Input: dimensioned drawing with shaded views. Units: mm. Origin: part minimum x, y, z. A direction names the side the tool comes from. Give positions to 0.01 mm unless a question says otherwise; leave off trailing zeros. Order: outer loops, then holes, each group sorted by start corner. A loop starts at its lowest first (then second) coordinate and runs counter-clockwise, first axis right, second up. Notation, with made-up numbers: (6, 11.5) - (16, 11.5) arc R29 cw to (16, 34.5) - close; hole circle Ø7 at (7.5, 47.25). An arc over 180 degrees is marked (long way). Answer as CSV lines item,"result".
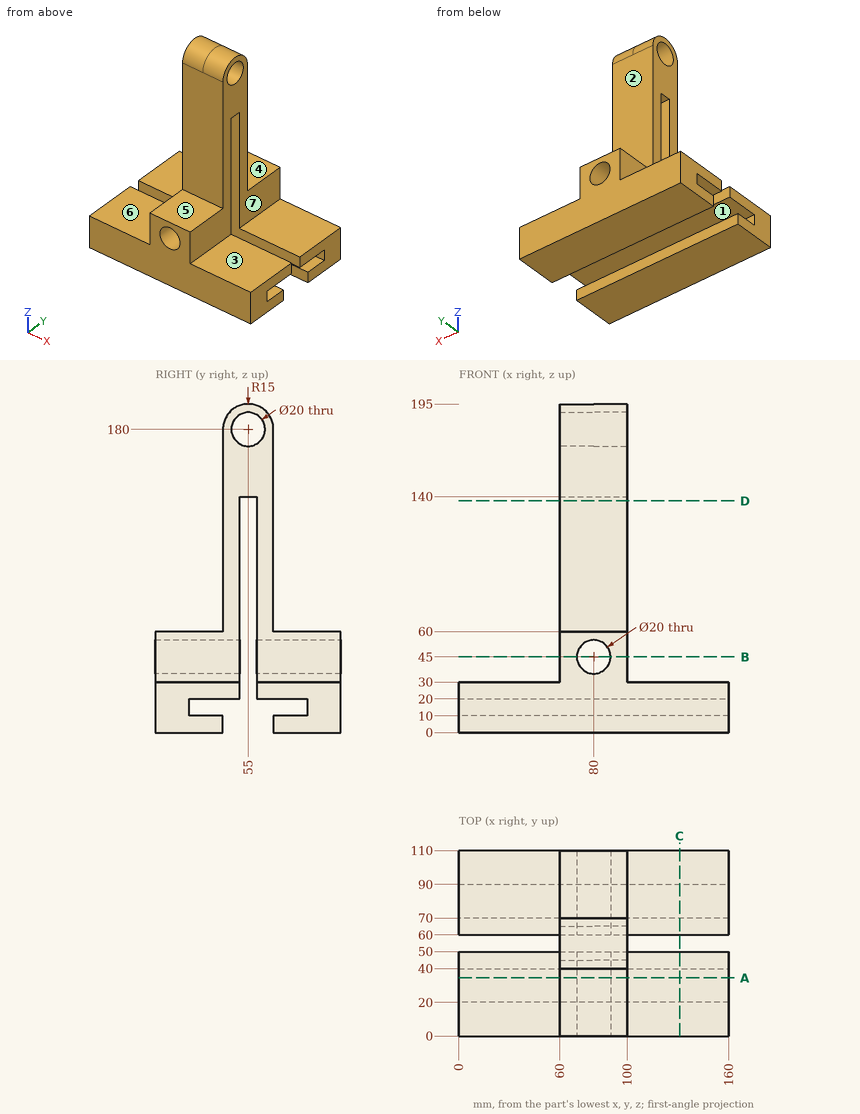
(1) Cut plane C-C (x = 131). Return loops of the section in (y, z).
Completed:
outline,"(0, 0) - (40, 0) - (40, 10) - (20, 10) - (20, 20) - (50, 20) - (50, 30) - (0, 30) - close; (60, 20) - (90, 20) - (90, 10) - (70, 10) - (70, 0) - (110, 0) - (110, 30) - (60, 30) - close"
(2) Cut plane D-D (z = 137.5). Return loops of the section in (x, y), then the cut area to 3 significant figures.
Completed:
outline,"(60, 40) - (100, 40) - (100, 50) - (60, 50) - close; (60, 60) - (100, 60) - (100, 70) - (60, 70) - close"
area,"800 mm²"
(3) Mould query, pull axis Y, two halves, no side actions, for the marked faces 1, 2 and 3. Classes: released by +Y, released by -Y, zero draft, split by the parting line, or undercut.
Completed:
face 1,"undercut"
face 2,"released by +Y"
face 3,"zero draft"
(4) Cut plane A-A (y = 34.5). Return loops of the section in (x, z).
Completed:
outline,"(0, 0) - (160, 0) - (160, 10) - (0, 10) - close; (0, 20) - (160, 20) - (160, 30) - (100, 30) - (100, 60) - (60, 60) - (60, 30) - (0, 30) - close; hole circle Ø20 at (80, 45)"
(5) Cut plane B-B (z = 45). Return loops of the section in (x, y), then the cut area to 3 significant figures.
Completed:
outline,"(60, 0) - (70, 0) - (70, 50) - (60, 50) - close; (60, 60) - (70, 60) - (70, 110) - (60, 110) - close; (90, 0) - (100, 0) - (100, 50) - (90, 50) - close; (90, 60) - (100, 60) - (100, 110) - (90, 110) - close"
area,"2,000 mm²"
(6) Access query for the marked faces 4, 5, 6 and 7. Directions: +Z, -Z, +X, -X, +Y, -Y. A direction counts if a zero-diameter tool reaches every point of the face in a straight line with its end or side. Return the directions, or none.
Completed:
face 4,"+Z, +X, -X, +Y"
face 5,"+Z, +X, -X, -Y"
face 6,"+Z, -X, +Y, -Y"
face 7,"+Z, +X, +Y, -Y"
(7) Contact query for flat-ended pins moving along their axis: pin 1 (3 mm diameter, centred on x = 59, y = 82, fed in from -Z); pin 2 (16 mm diameter, centred on y = 55, z = 180, fed in from +X); pin 3 (1.5 mm diameter, centred on x = 60, y = 74.5, fed in from +Z); pin 4 (8 mm diameter, centred on y = 42.5, z = 122.5, fed in from -X). Output: stop coordinate, or through.
Completed:
pin 1,"z = 0"
pin 2,"through"
pin 3,"z = 60"
pin 4,"x = 60"
(8) Ray query, line 1 (Z direction, x = 80, y = 89.5); line 2 (Z direction, x = 30, y = 22); line 3 (Y direction, x = 76, z = 180). Return the intervals inside material, ascending. Write a range as from..to.
Completed:
line 1,"0..10, 20..35, 55..60"
line 2,"0..10, 20..30"
line 3,"40..45, 65..70"
